Design review of the part built by this model. Coordinates are the model's own, in mm. Round coordinates to 2 decimals unless told otherwise and drop trailing zeros. Order: outer loops, then holes, each group sorted by start corner. A loop starts at its lowest first (then second) coordinate and runs counter-clockwise, first axis right, second up.
from build123d import *

# Parameters (mm, degrees)
SKETCH1_R           = 6.35
SKETCH1_R_2         = 3.175
BOSS_EXTRUDE1_DEPTH = 3.175


with BuildPart() as part:
    # Sketch1 → Boss-Extrude1 (new body)
    with BuildSketch(Plane(origin=(0, 0, 0), x_dir=(1, 0, 0), z_dir=(0, 1, 0))):
        Polygon((0, 0), (139.954, 0), (69.977, 121.203719361), align=None)
        with Locations((69.977, 40.401239787)):
            Circle(SKETCH1_R, mode=Mode.SUBTRACT)
        with Locations((117.956954744, 12.7)):
            Circle(SKETCH1_R_2, mode=Mode.SUBTRACT)
        with Locations((21.997045256, 12.7)):
            Circle(SKETCH1_R_2, mode=Mode.SUBTRACT)
        with Locations((69.977, 95.803719361)):
            Circle(SKETCH1_R_2, mode=Mode.SUBTRACT)
    extrude(amount=BOSS_EXTRUDE1_DEPTH)


solid = part.part
1) Take a section at D-D on z = -81. Give the boundary of the cut face in (x, y) (3 decimals).
Results:
outline: (46.765, 0) - (93.189, 0) - (93.189, 3.175) - (46.765, 3.175) - close
2) Take a section at C-C on x = 14.5. Give the boundary of the cut face in (y, z) (3 decimals).
Results:
outline: (0, -25.115) - (3.175, -25.115) - (3.175, 0) - (0, 0) - close
3) Take a section at A-A on y = 2.2. Give the boundary of the cut face in (x, z) (3 decimals).
Results:
outline: (0, 0) - (69.977, -121.204) - (139.954, 0) - close; hole circle Ø6.35 at (21.997, -12.7); hole circle Ø12.7 at (69.977, -40.401); hole circle Ø6.35 at (69.977, -95.804); hole circle Ø6.35 at (117.957, -12.7)
4) Clearance check with a flat-ended pin moving along its axis: P1, Ø1.5, axis at x = 109, y = 1.5, coming from the -Z side. State where the tip first meets the part, or that it passes through.
Results:
P1: stops at z = -54.91
5) To check wall thickness, follow line 1 along Z through (x, y) = (71, 1.4); line 2 along Z through (x, y) = (66, 2.4); line 3 along X through (y, z) = (2.2, -40). State the ranges of each line that lie inside material, in increasing order.
Results:
line 1: z = -119.43 to -98.81, -92.8 to -46.67, -34.13 to 0
line 2: z = -114.32 to -45.35, -35.45 to 0
line 3: x = 23.09 to 63.64, 76.31 to 116.86
6) The part is to be moulded in two halves that separate along X. For faces 1 (the face through (69, 0, -48)), 2 (the face through (114.785, 1.565, -12.84)), 3 (the face through (67.46, 1.57, -93.87)), 4 (the face through (105.455, 1.565, -59.753)), say which applies: released by +X, released by -X, zero draft, split by the parting line, or undercut.
Results:
face 1: zero draft
face 2: undercut
face 3: undercut
face 4: released by +X
7) Take a section at B-B on z = -12.7. Give the boundary of the cut face in (x, y) (3 decimals), plus the area to 3 significant figures.
Results:
outline: (7.332, 0) - (18.822, 0) - (18.822, 3.175) - (7.332, 3.175) - close; (25.172, 0) - (114.782, 0) - (114.782, 3.175) - (25.172, 3.175) - close; (121.132, 0) - (132.622, 0) - (132.622, 3.175) - (121.132, 3.175) - close
area: 357 mm2
